from build123d import *

# Parameters (mm, degrees)
F1_DEPTH = 2
F2_W     = 51.6000000954
F2_H     = 43.3000000954
F3_DEPTH = 3
F4_DEPTH = 17.9


with BuildPart() as f1:
    # F0 (on Top) → F1 (new body)
    with BuildSketch(Plane.XY):
        Polygon((-9.1260878563, 7.6790904999), (-64.9260878563, 7.6790904999), (-64.9260878563, -39.8209095001), (-9.1260878563, -39.8209095001), (-9.1260878563, -16.0709095001), align=None)
        with BuildLine():
            ThreePointArc((-50.9760878563, -9.1959095001), (-55.9760878563, -4.1959095001), (-50.9760878563, 0.8040904999))
            Line((-50.9760878563, 0.8040904999), (-23.0760878563, 0.8040904999))
            ThreePointArc((-23.0760878563, 0.8040904999), (-18.0760878563, -4.1959095001), (-23.0760878563, -9.1959095001))
            Line((-23.0760878563, -9.1959095001), (-50.9760878563, -9.1959095001))
        make_face(mode=Mode.SUBTRACT)
    extrude(amount=F1_DEPTH)

    # F2 (on face) → F3 (join)
    with BuildSketch(Plane(origin=(0, 0, 0), x_dir=(1, 0, 0), z_dir=(0, 0, -1))):
        with Locations((-37.0260878563, 16.0709095001)):
            Rectangle(F2_W, F2_H)
    extrude(amount=F3_DEPTH)

    # F4 (cut): a face of the model
    f4_faces = [f1.faces().sort_by_distance(p)[0] for p in [
        (-37.0260878563, -4.1959095001, 0),
    ]]
    extrude(f4_faces, amount=-F4_DEPTH, mode=Mode.SUBTRACT)


solid = f1.part
Part model, mm, in its own coordinate system. A direction names the side the tool comes from. Give positions to 0.01 mm unless a question says otherwise; leave off trailing zeros. Order: outer loops, then holes, each group sorted by start corner. A loop starts at its lowest first (then second) coordinate and runs counter-clockwise, first axis right, second up. Notation, with made-up numbers: (23.25, 9.25) - (34.25, 9.25) arc R13 cw to (34.25, 34.25) - close; hole circle Ø3 at (-12.75, 23). An arc over 180 degrees is marked (long way). One line per question, with ' | ' between items.
1. Pull direction X, two halves, no side cores. Call faces 1 (the face through (-39, -39, 0)), 2 (the face through (-9.126, -16, 1)), 3 (the face through (-18.077, -4.086, -0.465)): +X half, -X half, draft (parallel to the pull), parting line (faces both ways), or undercut.
Filled in:
face 1: draft | face 2: +X half | face 3: undercut
2. Drill centre lines: probe 1 along Y at (x, z) = (-41, -1.45); probe 2 along Y at (x, z) = (-43.5, 1.55); probe 3 along Y at (x, z) = (-62, -2.25). Where is each one in solid material? Low to high.
Filled in:
probe 1: -37.72 to -9.2, 0.8 to 5.58 | probe 2: -39.82 to -9.2, 0.8 to 7.68 | probe 3: -37.72 to 5.58
3. Band-saw the part on B-B on z = -1.85. List the corners of the cut face in (x, y).
Filled in:
outline: (-62.83, -37.72) - (-11.23, -37.72) - (-11.23, 5.58) - (-62.83, 5.58) - close; hole (-50.98, -9.2) - (-23.08, -9.2) arc R5 ccw to (-23.08, 0.8) - (-50.98, 0.8) arc R5 ccw to start
4. Band-saw the part on C-C on y = 3.5. List the corners of the cut face in (x, z).
Filled in:
outline: (-64.93, 0) - (-62.83, 0) - (-62.83, -3) - (-11.23, -3) - (-11.23, 0) - (-9.13, 0) - (-9.13, 2) - (-64.93, 2) - close
5. Band-saw the part on A-A on x = -45.5. List the corners of the cut face in (y, z).
Filled in:
outline: (-39.82, 0) - (-37.72, 0) - (-37.72, -3) - (-9.2, -3) - (-9.2, 2) - (-39.82, 2) - close; (0.8, -3) - (5.58, -3) - (5.58, 0) - (7.68, 0) - (7.68, 2) - (0.8, 2) - close
6. Band-saw the part on D-D on y = -6. List the corners of the cut face in (x, z).
Filled in:
outline: (-64.93, 0) - (-62.83, 0) - (-62.83, -3) - (-55.64, -3) - (-55.64, 2) - (-64.93, 2) - close; (-18.41, -3) - (-11.23, -3) - (-11.23, 0) - (-9.13, 0) - (-9.13, 2) - (-18.41, 2) - close
7. Drop flat-ended pins along their axis: P1, Ø1.5, axis at x = -38.5, z = -1.5, coming from the +Y side; P2, Ø2.5, axis at y = -21.5, z = -1.5, coming from the +X side. Give the stop position or say it passes through.
Filled in:
P1: y = 5.58 | P2: x = -11.23
8. Which spindle directions (+Z, -Z, +X, -X, +Y, -Y) get a long thin tool onto all of the face, cutting with end or side? Do faces 4 (the face through (-37, -37.721, -1)), 5 (the face through (-62.826, -16, -1)), 6 (the face through (-37, 0.804, 0)), 7 (the face through (-11.226, -16, -1)). Say none if no direction does.
Filled in:
face 4: -Z, +X, -X, -Y | face 5: -Z, -X, +Y, -Y | face 6: +Z, -Z | face 7: -Z, +X, +Y, -Y
